Here's how the part is built. I have some questions about the finished solid (model axes, mm). Face numbers are marked on the shaded views. A direction names the side the tool comes from. Coordinates: 2 decimals unless noted, no trailing zeros. Write each loop counter-clockwise with the first axis right and the second up, starting at its lowest first coordinate (ties: lowest second). Pieces come first, ordered by that corner, then holes.
Item 1: If we section it at B-B (z = 13): Please give me the cut outline in (x, y).
Item 2: If I drill on line 1 (Z direction, x = -18.5, y = 18); line 2 (X direction, y = 3, z = 24); line 3 (Y direction, x = -15.5, z = -13), over which ranges is the centre line in solid material (lowest first)?
Item 3: For the marked faces 1 and 2, which set-ups out of +Z, -Z, +X, -X, +Y, -Y let a thin tool reach every point of the face, with its end or its side?
Item 4: If we section it at A-A (y = 8): Please give me the cut outline in (x, z).
Item 5: If we section it at D-D (x = -12.5): Please give me the cut outline in (y, z), then the cut area to 3 significant figures.
Item 6: I'm going to push flat-ended pins straight in: pin 1 Ø10 at (x, z) = (-25, -11.5) entering from -Y; pin 2 Ø10 at (x, y) = (-22, -13) entering from +Z; pin 3 Ø2 at (y, z) = (15.5, 18) entering from -X; pin 4 Ø11.5 at (y, z) = (3.24, 17.35) entering from +X. Where does each tip first touch, or does it pass through?
Item 7: If we section it at C-C (y = -13.5): Please give me the cut outline in (x, z), then the cut area to 3 significant figures.
Item 8: We'd pull the mould along Y, two halves only. Please class the marked faces 3, 4, 5 and 6: +Y half, -Y half, draft (parallel to the pull), parting line (faces both ways), or undercut.
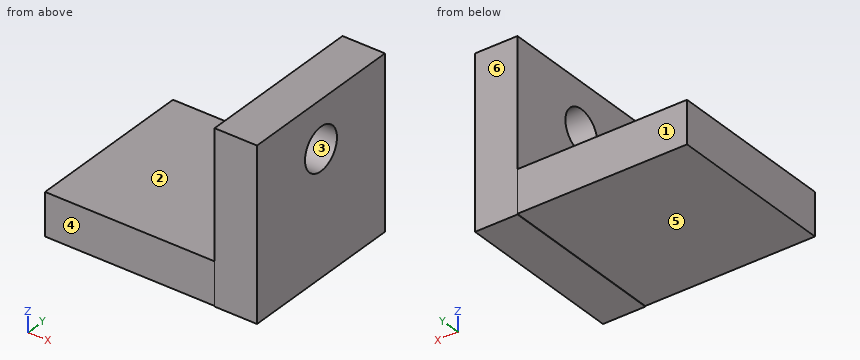
from build123d import *

# Parameters (mm, degrees)
F0_W     = 50.8
F0_H     = 50.8
F2_DEPTH = 12.7
F1_W     = 50.8
F1_H     = 12.7
F3_DEPTH = 50.8
F4_R     = 6.35
F5_DEPTH = 12.701


with BuildPart() as f2:
    # F0 (on Right) → F2 (new body)
    with BuildSketch(Plane.YZ):
        with Locations((3.236649, 6.020112)):
            Rectangle(F0_W, F0_H)
    extrude(amount=F2_DEPTH)

    # F1 (on Right) → F3 (join)
    with BuildSketch(Plane.YZ):
        with Locations((3.302505, -12.88737)):
            Rectangle(F1_W, F1_H)
    extrude(amount=-F3_DEPTH)

    # F4 (on Right) → F5 (cut, through all)
    with BuildSketch(Plane.YZ):
        with Locations((3.236649, 17.348448)):
            Circle(F4_R)
    extrude(amount=F5_DEPTH, mode=Mode.SUBTRACT)


solid = f2.part
Answer list:
1. outline: (0, -22.16) - (12.7, -22.16) - (12.7, -1.39) - (0, -1.39) - close; (0, 7.86) - (12.7, 7.86) - (12.7, 28.64) - (0, 28.64) - close
2. line 1: z = -19.24 to -6.54
2. line 2: x = 0 to 12.7
2. line 3: y = -22.1 to 28.7
3. face 1: +Z, -Z, +X, -X, +Y
3. face 2: +Z, -X, +Y, -Y
4. outline: (-50.8, -19.24) - (0, -19.24) - (0, -19.38) - (12.7, -19.38) - (12.7, 13.15) - (0, 13.15) - (0, -6.54) - (-50.8, -6.54) - close; (0, 21.55) - (12.7, 21.55) - (12.7, 31.42) - (0, 31.42) - close
5. outline: (-22.1, -19.24) - (28.7, -19.24) - (28.7, -6.54) - (-22.1, -6.54) - close
5. area: 645 mm2
6. pin 1: stops at y = -22.1
6. pin 2: stops at z = -6.54
6. pin 3: stops at x = 0
6. pin 4: passes through
7. outline: (-50.8, -19.24) - (0, -19.24) - (0, -19.38) - (12.7, -19.38) - (12.7, 31.42) - (0, 31.42) - (0, -6.54) - (-50.8, -6.54) - close
7. area: 1,290 mm2
8. face 3: undercut
8. face 4: -Y half
8. face 5: draft
8. face 6: +Y half
